Read the model definition and answer for the solid it produces. Units are mm, in the model's axes. A direction names the side the tool comes from. Give positions to 0.01 mm unless a question says otherwise; leave off trailing zeros. Loops run counter-clockwise (first coordinate to the right, second up) from the corner with the lowest first, then second, coordinate; pieces in that order, holes last.
(1) Find section D-D, the plane z = -0.75. Write down the section's boundary in (x, y).
(2) Straight lines are drawn through the part: probe 1 along Z at (x, y) = (1.25, -2.75); probe 2 along Y at (x, z) = (-1.5, 9); probe 3 along Y at (x, z) = (0.5, -2.5). For each, find the intervals that lie inside material, in ascending order.
(3) Which of the six approach directions +Z, -Z, +X, -X, +Y, -Y give full straight-line access (tool end or side, diameter ignored) to faces 1 (the face through (-1.5, -2.4, -9.85)), 2 (the face through (-2.44, -0.54, -0.13)), 3 (the face through (-2.44, -0.54, 10.54))?
(4) Determine the mould class of faces 4 (the face through (-1.5, -2.4, 9.25)), 5 (the face through (0, 0, 11.35)), 6 (the face through (0, 0, -11.35)) for opening direction Z: pulls with the +Z half, pulls with the -Z half, needs draft (parallel to the pull), parting line crosses it, or undercut.
(5) Find section A-A, the plane x = 2.75. Write down the section's boundary in (y, z), then the cut area to 3 significant figures.
(6) Each of these flat-tipped pins is pushed along its axis until it touches: P1, Ø1.5, axis at x = -2, z = 6, coming from the +Y side; P2, Ø2, axis at x = -1.5, z = 6, coming from the +Y side; P3, Ø2, axis at y = -3, z = 5, coming from the +X side. Where does it stop, or does it pass through?
Autodesk Inventor part; units mm, degrees
ref_plane "cd_XY" through (0, 0, 0) normal (1, 0, 0) x (0, 0, -1)
ref_plane "cd_YZ" through (0, 0, 0) normal (0, 0, -1) x (0, 1, 0)
ref_plane "cd_ZX" through (0, 0, 0) normal (0, 1, 0) x (1, 0, 0)
sketch "Sketch_1" plane through (0, 0, 0) normal (1, 0, 0) x (0, 1, 0)
  line L0 (0, -50) -> (0, 50)
  line L1 (0, 11.35) -> (2.4, 11.35)
  line L2 (2.4, 11.35) -> (2.5, 11.25)
  line L3 (2.5, 11.25) -> (2.5, 9.85)
  line L4 (2.5, 9.85) -> (2.4, 9.85)
  line L5 (2.4, 9.85) -> (2.4, 9.15)
  line L6 (2.4, 9.15) -> (2.5, 9.15)
  line L7 (2.5, 9.15) -> (2.5, -9.15)
  line L8 (2.5, -9.15) -> (2.4, -9.15)
  line L9 (2.4, -9.15) -> (2.4, -9.85)
  line L10 (2.4, -9.85) -> (2.5, -9.85)
  line L11 (2.5, -9.85) -> (2.5, -11.25)
  line L12 (2.5, -11.25) -> (2.4, -11.35)
  line L13 (2.4, -11.35) -> (0, -11.35)
  line L14 (0, -11.35) -> (0, 11.35)
revolve "Revolution1" add sketch "Sketch_1" angle 360 about axis through (0, 0, -50) along (0, 0, -1)
sketch "Sketch_4" plane through (0, 0, 9.85) normal (0, 0, 1) x (1, 0, 0)
  arc A0 (2, -2.248) -> (-2, -2.248) centre (0, 0.25) ccw
  line L0 (-2, -2.248) -> (-2, -4.75)
  line L1 (-2, -4.75) -> (2, -4.75)
  line L2 (2, -4.75) -> (2, -2.248)
extrude "Extrusion1" add sketch "Sketch_4" against normal blind 0.6
sketch "Sketch_5" plane through (0, 0, -9.85) normal (0, 0, 1) x (1, 0, 0)
  arc A0 (2, -2.248) -> (-2, -2.248) centre (0, 0.25) ccw
  line L0 (-2, -2.248) -> (-2, -4.75)
  line L1 (-2, -4.75) -> (2, -4.75)
  line L2 (2, -4.75) -> (2, -2.248)
extrude "Extrusion2" add sketch "Sketch_5" along normal blind 0.6
ref_plane "cd_XY" through (0, 0, 0) normal (1, 0, 0) x (0, 0, -1)
ref_plane "cd_YZ" through (0, 0, 0) normal (0, 0, -1) x (0, 1, 0)
ref_plane "cd_ZX" through (0, 0, 0) normal (0, 1, 0) x (1, 0, 0)
properties part number "CJ2-Z_CD-Z015"
Entries:
1. outline: circle Ø5 at (0, 0)
2. probe 1: z = -9.85 to -9.25, 9.25 to 9.85
2. probe 2: y = -2 to 2
2. probe 3: y = -2.45 to 2.45
3. face 1: -Z
3. face 2: none
3. face 3: +Z
4. face 4: undercut
4. face 5: pulls with the +Z half
4. face 6: pulls with the -Z half
5. outline: (-1.39, -9.85) - (1.89, -9.85) - (1.89, -9.25) - (-1.39, -9.25) - close; (-1.39, 9.25) - (1.89, 9.25) - (1.89, 9.85) - (-1.39, 9.85) - close
5. area: 3.93 mm2
6. P1: stops at y = 2.17
6. P2: stops at y = 2.45
6. P3: stops at x = 1.5
